from build123d import *

# Parameters (mm, degrees)
BOSS_EXTRUDE4_DEPTH = 7.5


with BuildPart() as part:
    # Sketch3 → Boss-Extrude4 (new, symmetric)
    with BuildSketch(Plane(origin=(0, 0, 0), x_dir=(1, 0, 0), z_dir=(0, 1, 0))):
        Polygon((-14, 0), (14, 0), (14, 5), (11, 5), (11, 2), (9, 2), (9, 5), (6, 5), (6, 2), (4, 2), (4, 5), (1, 5), (1, 2), (-1, 2), (-1, 5), (-4, 5), (-4, 2), (-6, 2), (-6, 5), (-9, 5), (-9, 2), (-11, 2), (-11, 5), (-14, 5), align=None)
    extrude(amount=BOSS_EXTRUDE4_DEPTH, both=True)


solid = part.part
Can you work these out from the model? Positions are in its coordinate system, mm. A direction names the side the tool comes from. Coordinates: 2 decimals unless noted, no trailing zeros. Loops run counter-clockwise (first coordinate to the right, second up) from the corner with the lowest first, then second, coordinate; pieces in that order, holes last. Notation, with made-up numbers: M 10,65.5 L 37,65.5 A13 ccw 37,74.5 Z; hole C -21,60 d5. An arc over 180 degrees is marked long. Answer as CSV lines item,"result". Start each with the question number.
1. For faces 1 (the face through (-12, 0, -5)), 2 (the face through (-6, 0, -3)), which set-ups out of +Z, -Z, +X, -X, +Y, -Y let a thin tool reach every point of the face, with its end or its side?
2. If I drill on probe 1 along X at (y, z) = (1, -2.45); probe 2 along Z at (x, y) = (9.75, -6), over which ranges is the centre line in solid material (lowest first)? Write a range as [from, to].
3. Suppose I cut it at B-B, the plane y = 2.5. List the corners of the cut face in (x, z) for me.
4. Thinking about a two-plate mould opening in X: for faces 3 (the face through (0, 7.5, -1)), 4 (the face through (14, 0, -2)), 5 (the face through (11, 0, -4)), which applies, +X half, -X half, draft (parallel to the pull), parting line (faces both ways), or undercut?
5. Suppose I cut it at A-A, the plane z = -3.7. List the corners of the cut face in (x, y) for me.
6. Suppose I cut it at C-C, the plane x = 5. List the corners of the cut face in (y, z) for me, plus the area to 3 significant figures.
7. For pin 1 Ø0.6 at (x, y) = (-10, 3) entering from -Z, with a flat end and sliding along its axis, tell me the tip position at first contact or that it passes through.
Output:
1,face 1,"-Z, +X, -X, +Y, -Y"
1,face 2,"-Z, +Y, -Y"
2,probe 1,"x = [-14, -11], [-9, -6], [-4, -1], [1, 4], [6, 9], [11, 14]"
2,probe 2,"z = [-2, 0]"
3,outline,"M -14,-5 L -11,-5 L -11,-2 L -9,-2 L -9,-5 L -6,-5 L -6,-2 L -4,-2 L -4,-5 L -1,-5 L -1,-2 L 1,-2 L 1,-5 L 4,-5 L 4,-2 L 6,-2 L 6,-5 L 9,-5 L 9,-2 L 11,-2 L 11,-5 L 14,-5 L 14,0 L -14,0 Z"
4,face 3,"draft"
4,face 4,"+X half"
4,face 5,"undercut"
5,outline,"M -14,-7.5 L -11,-7.5 L -11,7.5 L -14,7.5 Z; M -9,-7.5 L -6,-7.5 L -6,7.5 L -9,7.5 Z; M -4,-7.5 L -1,-7.5 L -1,7.5 L -4,7.5 Z; M 1,-7.5 L 4,-7.5 L 4,7.5 L 1,7.5 Z; M 6,-7.5 L 9,-7.5 L 9,7.5 L 6,7.5 Z; M 11,-7.5 L 14,-7.5 L 14,7.5 L 11,7.5 Z"
6,outline,"M -7.5,-2 L 7.5,-2 L 7.5,0 L -7.5,0 Z"
6,area,"30.0 mm^2"
7,pin 1,"stops at z = -2"
